Could you check a few things on this model? Use its own coordinates, in mm. A direction names the side the tool comes from. Give positions to 0.01 mm unless a question says otherwise; leave off trailing zeros. Order: outer loops, then holes, each group sorted by start corner. A loop starts at its lowest first (then second) coordinate and runs counter-clockwise, first axis right, second up. Notation, with made-up numbers: (-13, 49.5) - (44, 49.5) arc R7 cw to (44, 54.5) - close; hole circle Ø4 at (-12.75, -5.75). An arc over 180 degrees is marked (long way). Put each result on its own line as item: value.
from build123d import *

# Parameters (mm, degrees)
SKETCH_1_W          = 100
SKETCH_1_H          = 110
EXTRUDE_1_DEPTH     = 100
SKETCH_2_W          = 30
SKETCH_2_H          = 21
CUT_EXTRUDE_1_DEPTH = 100
EXTRUDE_START       = -100
EXTRUDE_3_DEPTH     = 100
EXTRUDE_2_DEPTH     = 4
EXTRUDE_3_2_DEPTH   = 4
SKETCH_4_W          = 6.1
SKETCH_4_H          = 11.5
CUT_EXTRUDE_4_DEPTH = 4
SKETCH_6_W          = 10
SKETCH_6_H          = 45.995714962
EXTRUDE_4_DEPTH     = 46
SKETCH_7_R          = 22.997857481
EXTRUDE_5_DEPTH     = 4
EXTRUDE_START_2     = 4
SKETCH_8_R          = 22.997857481
EXTRUDE_6_DEPTH     = 4


# Read off the part's stored shape, not the designer's step: 拉伸-薄壁3
with BuildPart() as part:
    # 草图1 → 凸台-拉伸1 (new body)
    with BuildSketch(Plane.XY):
        Polygon((-4, 0), (-4, 114), (104, 114), (104, -4), (-4, -4), align=None)
        with Locations((50, 55)):
            Rectangle(SKETCH_1_W, SKETCH_1_H, mode=Mode.SUBTRACT)
    extrude(amount=EXTRUDE_1_DEPTH)

    # 草图2 → 切除-拉伸1 (cut)
    with BuildSketch(Plane.XY.offset(100)):
        with Locations((11, 103.5)):
            Rectangle(SKETCH_2_W, SKETCH_2_H)
    cut_extrude_1 = extrude(amount=-CUT_EXTRUDE_1_DEPTH, mode=Mode.SUBTRACT)

    # Extrude 3 outline → Extrude 3 (add)
    with BuildSketch(Plane.XY.offset(100).offset(EXTRUDE_START)):
        Polygon((74, 110), (70, 110), (70, 89), (100, 89), (100, 93), (74, 93), align=None)
        Polygon((26, 93), (0, 93), (0, 89), (30, 89), (30, 110), (26, 110), align=None)
    extrude(amount=EXTRUDE_3_DEPTH)

    # 镜向1: 切除-拉伸1 across plane
    add(cut_extrude_1.mirror(Plane(origin=(50, 0, 0), x_dir=(0, 0, 1), z_dir=(1, 0, 0))), mode=Mode.SUBTRACT)

    # 草图3<3> → 凸台-拉伸2 (add)
    with BuildSketch(Plane.XY.offset(100)):
        Polygon((26, 93), (-4, 93), (-4, -4), (104, -4), (104, 93), (74, 93), (74, 114), (26, 114), align=None)
    extrude(amount=EXTRUDE_2_DEPTH)

    # 草图3<4> → Extrude 3 2 (add)
    with BuildSketch(Plane.XY.offset(100).offset(EXTRUDE_START)):
        Polygon((26, 93), (-4, 93), (-4, -4), (104, -4), (104, 93), (74, 93), (74, 114), (26, 114), align=None)
    extrude(amount=-EXTRUDE_3_2_DEPTH)

    # 草图4 → 切除-拉伸4 (cut)
    with BuildSketch(Plane(origin=(0, 114, 0), x_dir=(1, 0, 0), z_dir=(0, 1, 0))):
        with Locations((46.95, -44.25)):
            Rectangle(SKETCH_4_W, SKETCH_4_H)
        with Locations((53.05, -44.25)):
            Rectangle(SKETCH_4_W, SKETCH_4_H)
        with Locations((46.95, -55.75)):
            Rectangle(SKETCH_4_W, SKETCH_4_H)
        with Locations((53.05, -55.75)):
            Rectangle(SKETCH_4_W, SKETCH_4_H)
    extrude(amount=-CUT_EXTRUDE_4_DEPTH, mode=Mode.SUBTRACT)

    # 草图6 → 凸台-拉伸4 (add)
    with BuildSketch(Plane.XZ.offset(4)):
        with Locations((50.313928752, 50)):
            Rectangle(SKETCH_6_W, SKETCH_6_H)
    extrude(amount=EXTRUDE_4_DEPTH)

    # 草图7 → 凸台-拉伸5 (add)
    with BuildSketch(Plane(origin=(55.313928752, 0, 0), x_dir=(0, 0, -1), z_dir=(1, 0, 0))):
        with Locations((-50, -27)):
            Circle(SKETCH_7_R)
    extrude(amount=EXTRUDE_5_DEPTH)

    # 草图8 → 凸台-拉伸6 (add)
    with BuildSketch(Plane.ZY.offset(-45.313928752).offset(EXTRUDE_START_2)):
        with Locations(Location((50, -27, 0), (0, 0, 180))):
            Circle(SKETCH_8_R)
    extrude(amount=-EXTRUDE_6_DEPTH)


solid = part.part
1) Which directions (+Z, -Z, +X, -X, +Y, -Y) give clear straight access to the entire face, cutting with the end or side of a thin tool? Please do faces 1 (the flat face through (85, 89, 49)), 2 (the flat face through (50, -27, 72.998)), 3 (the flat face through (43.9, 112, 50)), 4 (the flat face through (55.314, -49.5, 56.7)).
Filled in:
face 1: none
face 2: +Z, +X, -X, -Y
face 3: +Y
face 4: +X, -Y
2) Suppose I cut it at B-B, the plane x = 88. List the corners of the cut face in (y, z) for me, and give its area (3 significant figures).
Filled in:
outline: (-4, -4) - (93, -4) - (93, 104) - (-4, 104) - close; hole (0, 0) - (89, 0) - (89, 100) - (0, 100) - close
area: 1,580 mm^2
3) Suppose I cut it at A-A, the plane y = 3. List the corners of the cut face in (x, z) for me.
Filled in:
outline: (-4, -4) - (104, -4) - (104, 104) - (-4, 104) - close; hole (0, 0) - (100, 0) - (100, 100) - (0, 100) - close
4) I'm going to push flat-ended pins straight in: pin 1 (14 mm diameter, centred on y = -29, z = 54, fed in from -X); pin 2 (4 mm diameter, centred on x = 25, z = 87, fed in from -Y); pin 3 (3 mm diameter, centred on x = 49, y = -38.5, fed in from +Z). Where does each tip first touch, or does it pass through?
Filled in:
pin 1: stops at x = 41.31
pin 2: stops at y = -4
pin 3: stops at z = 73
5) Suppose I cut it at D-D, the plane y = -35. List the corners of the cut face in (x, z) for me.
Filled in:
outline: (41.31, 28.44) - (45.31, 28.44) - (45.31, 27) - (55.31, 27) - (55.31, 28.44) - (59.31, 28.44) - (59.31, 71.56) - (55.31, 71.56) - (55.31, 73) - (45.31, 73) - (45.31, 71.56) - (41.31, 71.56) - close
6) If I drill on line 1 (Y direction, x = 46.5, z = 67.5); line 2 (X direction, y = 19, z = 12.5); line 3 (Y direction, x = 37, z = 9.5), over which ranges is the centre line in solid material (lowest first)? Write a range as [from, to].
Filled in:
line 1: y = [-50, 0], [110, 114]
line 2: x = [-4, 0], [100, 104]
line 3: y = [-4, 0], [110, 114]
7) We'd pull the mould along Y, two halves only. Please class faces 5 (the flat face through (49, 44, 100)), 6 (the flat face through (-4, 45, 51)): pulls with the +Y half, pulls with the -Y half, needs draft (parallel to the pull), parting line crosses it, or undercut.
Filled in:
face 5: undercut
face 6: needs draft
8) Suppose I cut it at C-C, the plane z = 13. List the corners of the cut face in (x, y) for me, and give its area (3 significant figures).
Filled in:
outline: (-4, -4) - (104, -4) - (104, 93) - (74, 93) - (74, 114) - (26, 114) - (26, 93) - (-4, 93) - close; hole (0, 0) - (100, 0) - (100, 89) - (70, 89) - (70, 110) - (30, 110) - (30, 89) - (0, 89) - close
area: 1,740 mm^2
